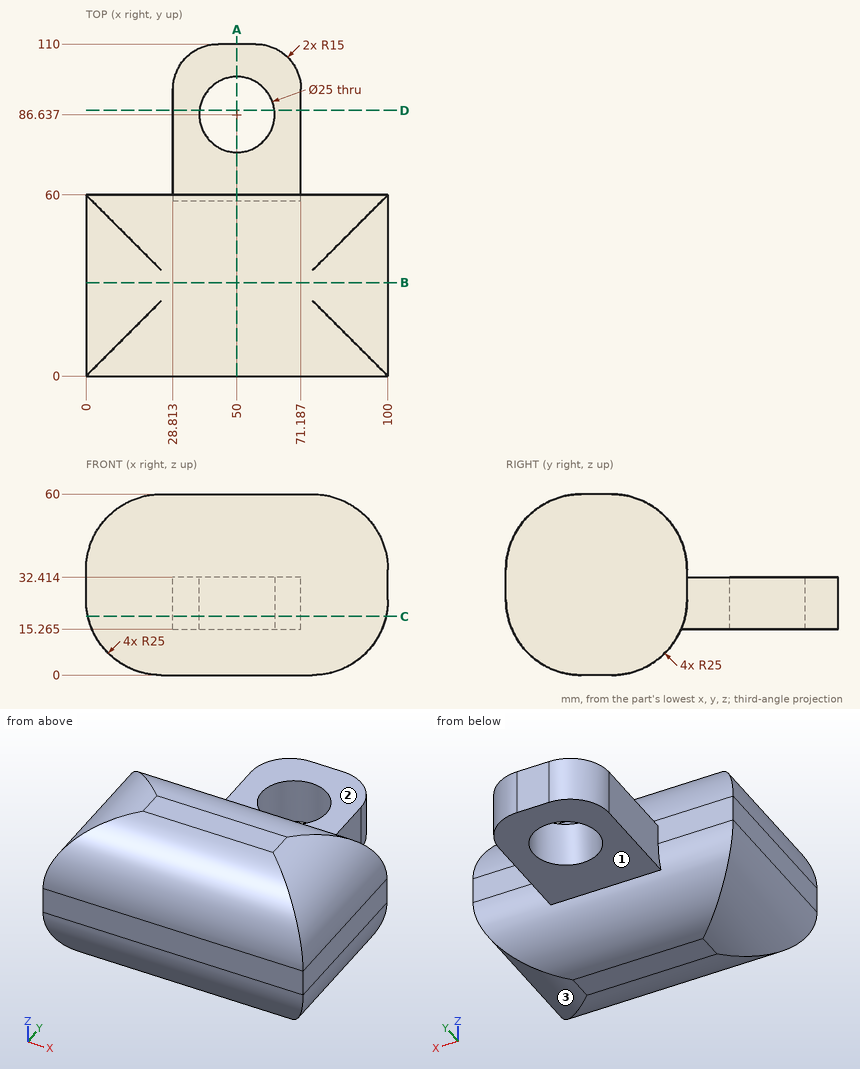
Answer from the drawing. Dimensions are ordinates in mm from the lowest x, y and z of the part. A direction names the side the tool comes from. Give positions to 0.01 mm unless a question says otherwise; leave off trailing zeros. Order: outer loops, then holes, each group sorted by start corner. A loop starts at its lowest first (then second) coordinate and runs counter-clockwise, first axis right, second up. Notation, with made-up numbers: (-26, -19.5) - (6, -19.5) arc R24 cw to (6, 17.5) - close; hole circle Ø10 at (-21, -1). An arc over 180 degrees is marked (long way). One line per item, written item: value. Start each with the question number.
1. Section B-B, the plane y = 31 is taken. Write down the section's boundary in (x, z), then the cut area to 3 significant figures.
2. Section C-C, the plane z = 19.5 is taken. Write down the section's boundary in (x, y), then the cut area to 3 significant figures.
3. Each of these flat-tipped pins is pushed along its axis until it touches: pin 1 Ø5 at (y, z) = (74.5, 26) entering from -X; pin 2 Ø6 at (x, z) = (14.5, 44) entering from -Y; pin 3 Ø1 at (y, z) = (35.5, 23.5) entering from -X. Where does it stop, or does it pass through?
4. Which of the six approach directions +Z, -Z, +X, -X, +Y, -Y give full straight-line access (tool end or side, diameter ignored) to the marked faces 1, 2 and 3?
5. Section A-A, the plane x = 50 is taken. Write down the section's boundary in (y, z) (1 decimal).
6. Section D-D, the plane y = 88 is taken. Write down the section's boundary in (x, z) (1 decimal).
7. Consider line 1 (Y direction, x = 50, z = 25.5); line 2 (X direction, y = 70, z = 16.5); line 3 (Y direction, x = 48, z = 35.5) (1 decimal). Determine where each line is inside the solid, lowest interval first.
Filled sheet:
1. outline: (0, 25) arc R25 ccw to (25, 0) - (75, 0) arc R25 ccw to (100, 25) - (100, 35) arc R25 ccw to (75, 60) - (25, 60) arc R25 ccw to (0, 35) - close
1. area: 5,460 mm²
2. outline: (0.61, 0.61) - (99.39, 0.61) - (99.39, 59.39) - (71.19, 59.39) - (71.19, 95) arc R15 ccw to (56.19, 110) - (43.81, 110) arc R15 ccw to (28.81, 95) - (28.81, 59.39) - (0.61, 59.39) - close; hole circle Ø25 at (50, 86.64)
2. area: 7,360 mm²
3. pin 1: x = 28.81
3. pin 2: y = 0.73
3. pin 3: x = 0.02
4. face 1: -Z, +X, -X, +Y
4. face 2: +Z, +X, -X, +Y
4. face 3: -Z, +X, +Y, -Y
5. outline: (0, 25) arc R25 ccw to (25, 0) - (35, 0) arc R25 ccw to (58, 15.3) - (74.1, 15.3) - (74.1, 32.4) - (60, 32.4) - (60, 35) arc R25 ccw to (35, 60) - (25, 60) arc R25 ccw to (0, 35) - close; (99.1, 15.3) - (110, 15.3) - (110, 32.4) - (99.1, 32.4) - close
6. outline: (28.8, 15.3) - (37.6, 15.3) - (37.6, 32.4) - (28.8, 32.4) - close; (62.4, 15.3) - (71.2, 15.3) - (71.2, 32.4) - (62.4, 32.4) - close
7. line 1: 0 to 74.14, 99.14 to 110
7. line 2: 28.81 to 71.19
7. line 3: 0 to 60
